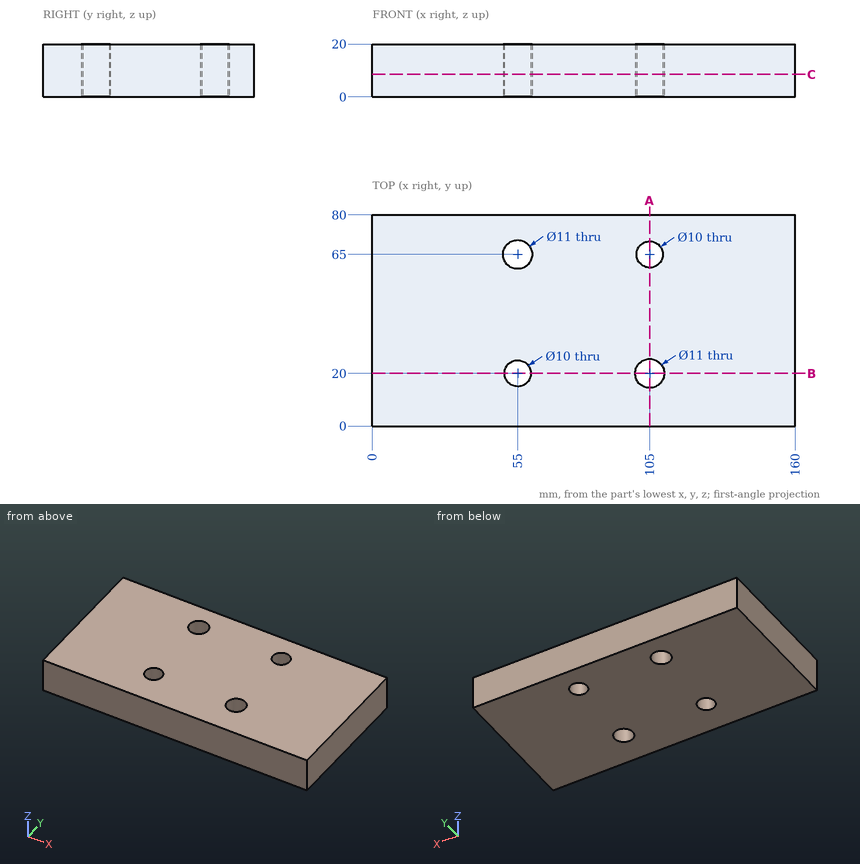
Can you work these out from the drawing? Everything is in mm from the part's minimum corner. Give positions to 0.01 mm unless a question says otherwise; leave off trailing zeros. Write each loop counter-clockwise with the first axis right and the second up, starting at its lowest first coordinate (ties: lowest second). Pieces come first, ordered by that corner, then holes. Notation, with made-up numbers: (31.5, -23.75) -> (59.5, -23.75) arc R28 ccw to (59.5, 2.25) -> close; hole circle Ø5 at (36.5, 68). An arc over 180 degrees is marked (long way). Write each question's results on one line, items separated by ' | '. Start each with the question number.
Q1. Suppose I cut it at A-A, the plane x = 105. List the corners of the cut face in (y, z) for me.
Q2. Suppose I cut it at C-C, the plane z = 8.5. List the corners of the cut face in (x, y) for me.
Q3. I need wall thicknesses on probe 1 along Y at (x, z) = (105, 13.75); probe 2 along Y at (x, z) = (55, 9.5); probe 3 along X at (y, z) = (24.5, 9.5). Which ranges of each line are inside material? Lowest first, please.
Q4. Suppose I cut it at B-B, the plane y = 20. List the corners of the cut face in (x, z) for me, and give its area (3 significant figures).
Q5. I'm going to push flat-ended pins straight in: pin 1 Ø6 at (x, y) = (105, 65) entering from +Z; pin 2 Ø3 at (y, z) = (13, 18) entering from -X. Where does each tip first touch, or does it pass through?
Outcome:
1) outline: (0, 0) -> (14.5, 0) -> (14.5, 20) -> (0, 20) -> close; (25.5, 0) -> (60, 0) -> (60, 20) -> (25.5, 20) -> close; (70, 0) -> (80, 0) -> (80, 20) -> (70, 20) -> close
2) outline: (0, 0) -> (160, 0) -> (160, 80) -> (0, 80) -> close; hole circle Ø11 at (55, 65); hole circle Ø10 at (55, 20); hole circle Ø11 at (105, 20); hole circle Ø10 at (105, 65)
3) probe 1: 0 to 14.5, 25.5 to 60, 70 to 80 | probe 2: 0 to 15, 25 to 59.5, 70.5 to 80 | probe 3: 0 to 52.82, 57.18 to 101.84, 108.16 to 160
4) outline: (0, 0) -> (50, 0) -> (50, 20) -> (0, 20) -> close; (60, 0) -> (99.5, 0) -> (99.5, 20) -> (60, 20) -> close; (110.5, 0) -> (160, 0) -> (160, 20) -> (110.5, 20) -> close | area: 2,780 mm2
5) pin 1: through | pin 2: x = 0
